Part print with two shaded views. Sizes in mm from the minimum x, y, z corner. A direction names the side the tool comes from. Coordinates: 2 decimals unless noted, no trailing zeros. Order: outer loops, then holes, each group sorted by start corner. A loop starts at its lowest first (then second) coordinate and runs counter-clockwise, first axis right, second up. Notation, with made-up numbers: (14.5, 21) - (29.5, 21) arc R22 ccw to (29.5, 50) - close; hole circle Ø11 at (18, 32). An arc over 180 degrees is marked (long way). Return JSON: item names as keys, results as strings.
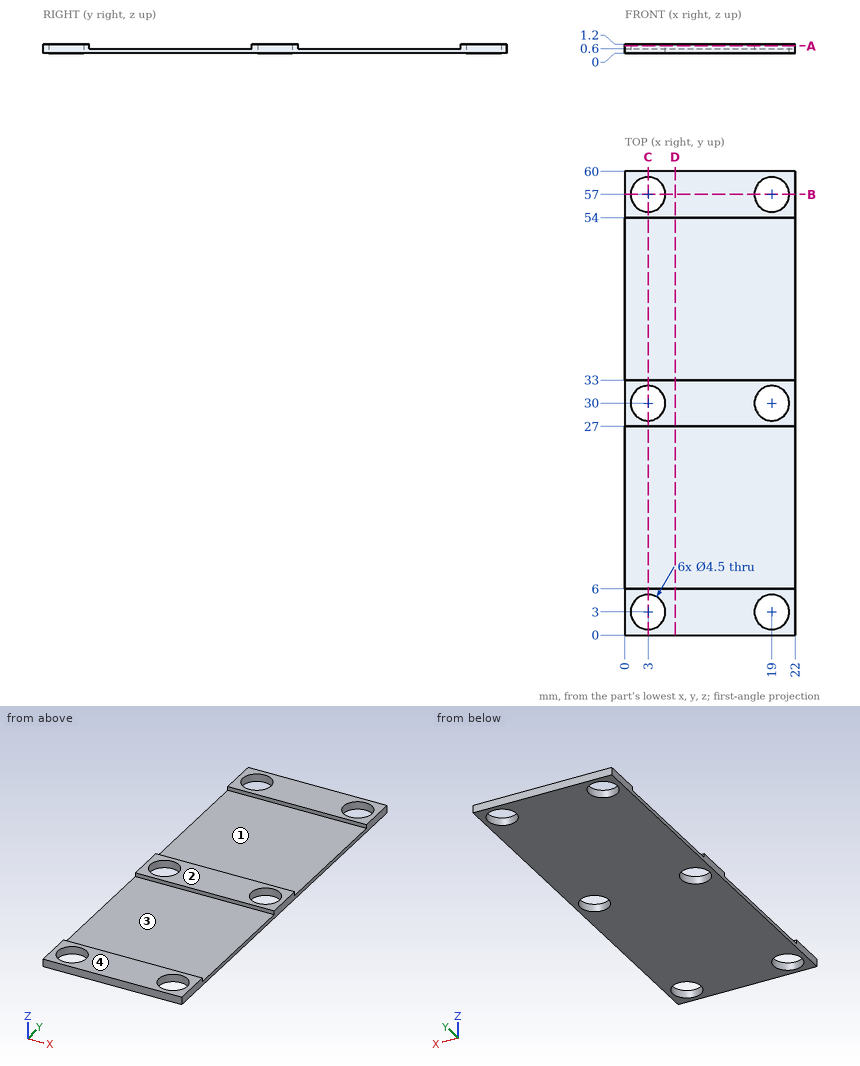
Item 1: Band-saw the part on C-C, the plane x = 3. List the corners of the cut face in (y, z).
Findings below:
{"outline": "(0, 0) - (0.75, 0) - (0.75, 1.2) - (0, 1.2) - close; (5.25, 0) - (27.75, 0) - (27.75, 1.2) - (27, 1.2) - (27, 0.6) - (6, 0.6) - (6, 1.2) - (5.25, 1.2) - close; (32.25, 0) - (54.75, 0) - (54.75, 1.2) - (54, 1.2) - (54, 0.6) - (33, 0.6) - (33, 1.2) - (32.25, 1.2) - close; (59.25, 0) - (60, 0) - (60, 1.2) - (59.25, 1.2) - close"}
Item 2: Drop a flat-ended pin along its axis: P1, Ø6.5, axis at x = 15, y = 39.5, coming from the +Z side. Give the stop position or say it passes through.
Findings below:
{"P1": "stops at z = 0.6"}
Item 3: Band-saw the part on A-A, the plane z = 0.95. Count the separate pieces of the cut face and the enclosed holes in it, then the cut area to 3 significant figures.
Findings below:
{"separate pieces": "3", "enclosed holes": "6", "area": "301 mm²"}
Item 4: Band-saw the part on D-D, the plane x = 6.5. List the corners of the cut face in (y, z), then the cut area to 3 significant figures.
Findings below:
{"outline": "(0, 0) - (60, 0) - (60, 1.2) - (54, 1.2) - (54, 0.6) - (33, 0.6) - (33, 1.2) - (27, 1.2) - (27, 0.6) - (6, 0.6) - (6, 1.2) - (0, 1.2) - close", "area": "46.8 mm²"}
Item 5: Band-saw the part on B-B, the plane y = 57. List the corners of the cut face in (x, z).
Findings below:
{"outline": "(0, 0) - (0.75, 0) - (0.75, 1.2) - (0, 1.2) - close; (5.25, 0) - (16.75, 0) - (16.75, 1.2) - (5.25, 1.2) - close; (21.25, 0) - (22, 0) - (22, 1.2) - (21.25, 1.2) - close"}
Item 6: Wall check: L1, parallel to Y at x = 14.75, z = 1.15; L2, parallel to Y at x = 19, z = 0.25; L3, parallel to Y at x = 3, z = 1. Give the ranges that are in metal, low to high. Write a range as [from, to].
Findings below:
{"L1": "y = [0, 6], [27, 33], [54, 60]", "L2": "y = [0, 0.75], [5.25, 27.75], [32.25, 54.75], [59.25, 60]", "L3": "y = [0, 0.75], [5.25, 6], [27, 27.75], [32.25, 33], [54, 54.75], [59.25, 60]"}
Item 7: Mould opens along Y. For the marked faces 3 and 4 say: released by +Y, released by -Y, zero draft, split by the parting line, or undercut.
Findings below:
{"face 3": "undercut", "face 4": "zero draft"}
Item 8: Which spindle directions (+Z, -Z, +X, -X, +Y, -Y) get a long thin tool onto all of the face, cutting with end or side? Do the marked faces 1 and 2. Say none if no direction does.
Findings below:
{"face 1": "+Z, +X, -X", "face 2": "+Z, +X, -X, +Y, -Y"}
